Part model, mm, in its own coordinate system. Round coordinates to 2 decimals unless told otherwise and drop trailing zeros. Loops run counter-clockwise (first coordinate to the right, second up) from the corner with the lowest first, then second, coordinate; pieces in that order, holes last.
from build123d import *

# Parameters (mm, degrees)
F0_W     = 155.575
F0_H     = 174.625
F0_W_2   = 79.375
F0_H_2   = 76.2
F1_DEPTH = 1.1811
F3_DEPTH = 1.1811
F4_R     = 2.54
F5_DEPTH = 1.1811
F6_R     = 5.08


with BuildPart() as f1:
    # F0 (on Top) → F1 (new body)
    with BuildSketch(Plane.XY):
        with Locations((0, 87.3125)):
            Rectangle(F0_W, F0_H)
        with Locations((-117.475, 87.3125)):
            Rectangle(F0_W_2, F0_H)
        with Locations((117.475, 87.3125)):
            Rectangle(F0_W_2, F0_H)
        with Locations((0, 212.725)):
            Rectangle(F0_W, F0_H_2)
    extrude(amount=F1_DEPTH)

    # F2 (on face) → F3 (cut, through all)
    with BuildSketch(Plane.XY.offset(1.1811)):
        with BuildLine():
            Line((33.3375, 0), (33.3375, 106.3625))
            ThreePointArc((33.3375, 106.3625), (0, 139.7), (-33.3375, 106.3625))
            Line((-33.3375, 106.3625), (-33.3375, 0))
            Line((-33.3375, 0), (33.3375, 0))
        make_face()
        with BuildLine():
            ThreePointArc((-52.7812, 250.825), (-57.15, 255.1938), (-61.5188, 250.825))
            Line((-61.5188, 250.825), (-61.5188, 192.0875))
            ThreePointArc((-61.5188, 192.0875), (-57.15, 187.7187), (-52.7812, 192.0875))
            Line((-52.7812, 192.0875), (-52.7812, 250.825))
        make_face()
        with BuildLine():
            ThreePointArc((61.5188, 250.825), (57.15, 255.1938), (52.7812, 250.825))
            Line((52.7812, 250.825), (52.7812, 192.0875))
            ThreePointArc((52.7812, 192.0875), (57.15, 187.7187), (61.5188, 192.0875))
            Line((61.5188, 192.0875), (61.5188, 250.825))
        make_face()
    extrude(amount=-F3_DEPTH, mode=Mode.SUBTRACT)

    # F4 (on face) → F5 (cut, through all)
    with BuildSketch(Plane.XY.offset(1.1811)):
        with BuildLine():
            ThreePointArc((-76.2, 155.575), (-77.7875, 157.1625), (-79.375, 155.575))
            Line((-79.375, 155.575), (-79.375, 136.525))
            ThreePointArc((-79.375, 136.525), (-77.7875, 134.9375), (-76.2, 136.525))
            Line((-76.2, 136.525), (-76.2, 155.575))
        make_face()
        with BuildLine():
            ThreePointArc((-76.2, 116.713), (-77.7875, 118.3005), (-79.375, 116.713))
            Line((-79.375, 116.713), (-79.375, 97.663))
            ThreePointArc((-79.375, 97.663), (-77.7875, 96.0755), (-76.2, 97.663))
            Line((-76.2, 97.663), (-76.2, 116.713))
        make_face()
        with BuildLine():
            ThreePointArc((-76.2, 77.851), (-77.7875, 79.4385), (-79.375, 77.851))
            Line((-79.375, 77.851), (-79.375, 58.801))
            ThreePointArc((-79.375, 58.801), (-77.7875, 57.2135), (-76.2, 58.801))
            Line((-76.2, 58.801), (-76.2, 77.851))
        make_face()
        with BuildLine():
            ThreePointArc((-76.2, 38.989), (-77.7875, 40.5765), (-79.375, 38.989))
            Line((-79.375, 38.989), (-79.375, 19.939))
            ThreePointArc((-79.375, 19.939), (-77.7875, 18.3515), (-76.2, 19.939))
            Line((-76.2, 19.939), (-76.2, 38.989))
        make_face()
        with BuildLine():
            Line((79.375, 136.525), (79.375, 155.575))
            ThreePointArc((79.375, 155.575), (77.7875, 157.1625), (76.2, 155.575))
            Line((76.2, 155.575), (76.2, 136.525))
            ThreePointArc((76.2, 136.525), (77.7875, 134.9375), (79.375, 136.525))
        make_face()
        with BuildLine():
            Line((79.375, 97.663), (79.375, 116.713))
            ThreePointArc((79.375, 116.713), (77.7875, 118.3005), (76.2, 116.713))
            Line((76.2, 116.713), (76.2, 97.663))
            ThreePointArc((76.2, 97.663), (77.7875, 96.0755), (79.375, 97.663))
        make_face()
        with BuildLine():
            Line((76.2, 77.851), (76.2, 58.801))
            ThreePointArc((76.2, 58.801), (77.7875, 57.2135), (79.375, 58.801))
            Line((79.375, 58.801), (79.375, 77.851))
            ThreePointArc((79.375, 77.851), (77.7875, 79.4385), (76.2, 77.851))
        make_face()
        with BuildLine():
            Line((79.375, 19.939), (79.375, 38.989))
            ThreePointArc((79.375, 38.989), (77.7875, 40.5765), (76.2, 38.989))
            Line((76.2, 38.989), (76.2, 19.939))
            ThreePointArc((76.2, 19.939), (77.7875, 18.3515), (79.375, 19.939))
        make_face()
        with BuildLine():
            ThreePointArc((-58.7375, 176.2125), (-60.325, 174.625), (-58.7375, 173.0375))
            Line((-58.7375, 173.0375), (-45.24375, 173.0375))
            ThreePointArc((-45.24375, 173.0375), (-43.65625, 174.625), (-45.24375, 176.2125))
            Line((-45.24375, 176.2125), (-58.7375, 176.2125))
        make_face()
        with BuildLine():
            ThreePointArc((-26.19375, 176.2125), (-27.78125, 174.625), (-26.19375, 173.0375))
            Line((-26.19375, 173.0375), (-12.7, 173.0375))
            ThreePointArc((-12.7, 173.0375), (-11.1125, 174.625), (-12.7, 176.2125))
            Line((-12.7, 176.2125), (-26.19375, 176.2125))
        make_face()
        with BuildLine():
            ThreePointArc((12.7, 176.2125), (11.1125, 174.625), (12.7, 173.0375))
            Line((12.7, 173.0375), (26.19375, 173.0375))
            ThreePointArc((26.19375, 173.0375), (27.78125, 174.625), (26.19375, 176.2125))
            Line((26.19375, 176.2125), (12.7, 176.2125))
        make_face()
        with BuildLine():
            ThreePointArc((45.24375, 176.2125), (43.65625, 174.625), (45.24375, 173.0375))
            Line((45.24375, 173.0375), (58.7375, 173.0375))
            ThreePointArc((58.7375, 173.0375), (60.325, 174.625), (58.7375, 176.2125))
            Line((58.7375, 176.2125), (45.24375, 176.2125))
        make_face()
        with Locations((-77.7875, 174.625)):
            Circle(F4_R)
        with Locations((77.7875, 174.625)):
            Circle(F4_R)
    extrude(amount=-F5_DEPTH, mode=Mode.SUBTRACT)

    # F6
    f6_edges = [f1.edges().sort_by_distance(p)[0] for p in [
        (-157.1625, 174.625, 0.59055),
        (-61.5188, 250.825, 0.59055),
        (-52.7812, 250.825, 0.59055),
        (52.7812, 250.825, 0.59055),
        (61.5188, 250.825, 0.59055),
        (157.1625, 174.625, 0.59055),
        (-157.1625, 0, 0.59055),
        (33.3375, 0, 0.59055),
        (-33.3375, 0, 0.59055),
        (157.1625, 0, 0.59055),
    ]]
    fillet(f6_edges, radius=F6_R)


solid = f1.part
1) Slice it at B-B, the plane y = 198. Give the cut face in (x, z).
Values:
outline: (-77.79, 0) - (-61.52, 0) - (-61.52, 1.18) - (-77.79, 1.18) - close; (-52.78, 0) - (52.78, 0) - (52.78, 1.18) - (-52.78, 1.18) - close; (61.52, 0) - (77.79, 0) - (77.79, 1.18) - (61.52, 1.18) - close
2) Drop a flat-ended pin along its axis: pin 1 Ø0.6 at (y, z) = (226, 0.5) entering from +X. Give the stop position or say it passes through.
Values:
pin 1: stops at x = 77.79
3) Slice it at A-A, the plane y = 86.5. Give the cut face in (x, z), then the cut area to 4 significant figures.
Values:
outline: (-157.16, 0) - (-33.34, 0) - (-33.34, 1.18) - (-157.16, 1.18) - close; (33.34, 0) - (157.16, 0) - (157.16, 1.18) - (33.34, 1.18) - close
area: 292.5 mm2
4) Slice it at D-D, the plane z = 0.4. Give the number of separate pieces and of enclosed holes in the cut face, then the cut area to 3 significant figures.
Values:
separate pieces: 1
enclosed holes: 12
area: 56,000 mm2
5) Mould opens along X. For faces 1 (the face through (0.733, 139.692, 0.599)), 2 (the face through (-37, 127, 0)) say: released by +X, released by -X, zero draft, split by the parting line, or undercut.
Values:
face 1: undercut
face 2: zero draft
6) Wall check: line 1 along X through (y, z) = (26.5, 0.85) (1 decimal); line 2 along X through (y, z) = (58.5, 0.25); line 3 along X through (y, z) = (90.5, 0.6). Give the ranges that are in metal, low to high.
Values:
line 1: x = -157.2 to -79.4, -76.2 to -33.3, 33.3 to 76.2, 79.4 to 157.2
line 2: x = -157.16 to -79.35, -76.23 to -33.34, 33.34 to 76.23, 79.35 to 157.16
line 3: x = -157.16 to -33.34, 33.34 to 157.16
7) Slice it at C-C, the plane x = 21. Give the cut face in (y, z) (1 decimal).
Values:
outline: (132.3, 0) - (173, 0) - (173, 1.2) - (132.3, 1.2) - close; (176.2, 0) - (250.8, 0) - (250.8, 1.2) - (176.2, 1.2) - close
